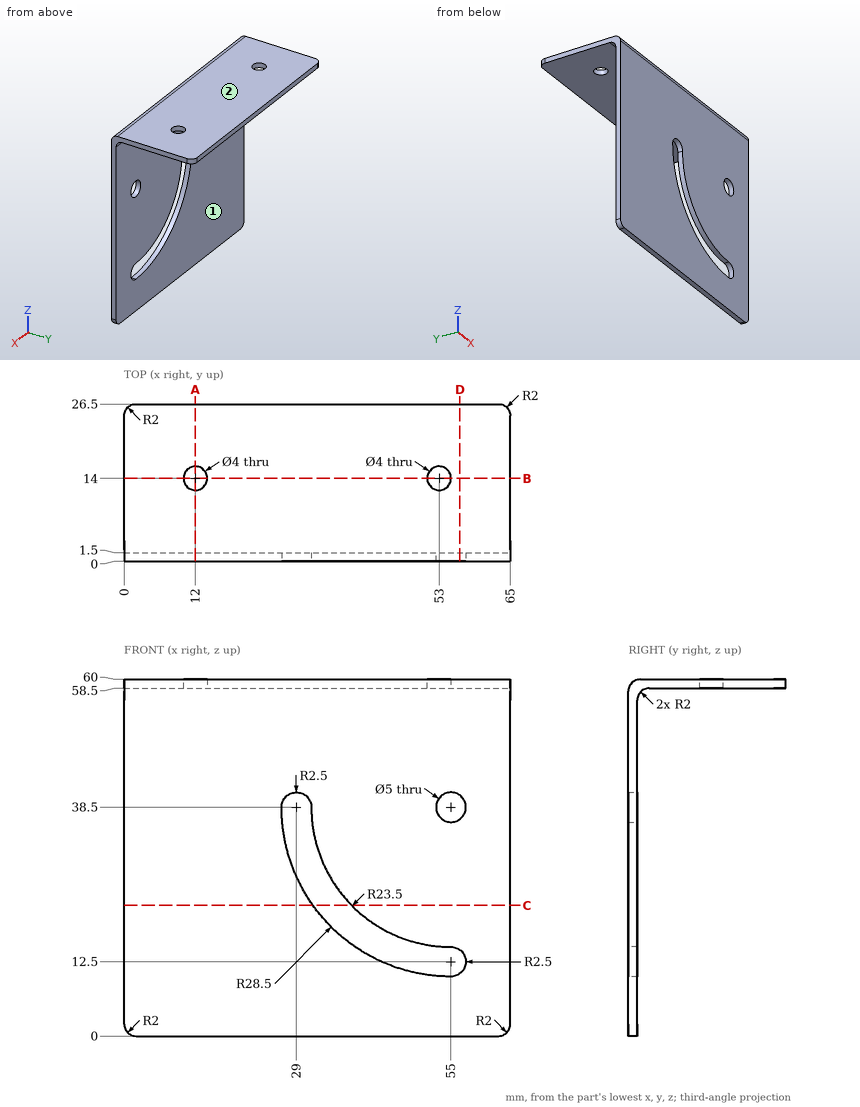
Verification items for this drawing (mm, ordinates from the low corner). A direction names the side the tool comes from. Coordinates: 2 decimals unless noted, no trailing zeros. Order: outer loops, then holes, each group sorted by start corner. A loop starts at its lowest first (then second) coordinate and runs counter-clockwise, first axis right, second up. Notation, with made-up numbers: (-23.5, 45.5) -> (26.5, 45.5) arc R15 cw to (26.5, 56.5) -> close; hole circle Ø3 at (47, -32). An arc over 180 degrees is marked (long way). Put each result on its own line as item: value. Start each with the question number.
1. Cross-section at B-B, the plane y = 14. Record the boundary of the cut face in (x, z).
2. Cross-section at C-C, the plane z = 22. Record the boundary of the cut face in (x, y), then the cut area to 3 significant figures.
3. Material ranges on L1, parallel to Z at x = 53, y = 10; L2, parallel to Y at x = 54, z = 7.5; L3, parallel to Z at x = 55, y = 0.9, recorded low to high. Write a range as [from, to].
4. Cross-section at D-D, the plane x = 56.5. Record the boundary of the cut face in (y, z).
5. Access from +Z, -Z, +X, -X, +Y, -Y to the whole of each face (thin tool, end or side, straight path). Record for the marked faces 1 and 2.
6. Go/stop test with flat-tipped pins: pin 1 Ø4 at (x, z) = (55, 38.5) entering from +Y; pin 2 Ø11.5 at (x, y) = (21, 11.5) entering from -Z. Record where each tip stops, or that it passes through.
7. Cross-section at A-A, the plane x = 12. Record the boundary of the cut face in (y, z).
Computed:
1. outline: (0, 58.5) -> (10, 58.5) -> (10, 60) -> (0, 60) -> close; (14, 58.5) -> (51, 58.5) -> (51, 60) -> (14, 60) -> close; (55, 58.5) -> (65, 58.5) -> (65, 60) -> (55, 60) -> close
2. outline: (0, 0) -> (31.76, 0) -> (31.76, 1.5) -> (0, 1.5) -> close; (38.27, 0) -> (65, 0) -> (65, 1.5) -> (38.27, 1.5) -> close
2. area: 87.7 mm2
3. L1: [58.5, 60]
3. L2: [0, 1.5]
3. L3: [0, 10], [15, 36], [41, 59.67]
4. outline: (0, 0) -> (1.5, 0) -> (1.5, 10.5) -> (0, 10.5) -> close; (0, 14.5) -> (1.5, 14.5) -> (1.5, 36.5) -> (0, 36.5) -> close; (0, 40.5) -> (1.5, 40.5) -> (1.5, 56.5) arc R2 cw to (3.5, 58.5) -> (26.5, 58.5) -> (26.5, 60) -> (2, 60) arc R2 ccw to (0, 58) -> close
5. face 1: -Z, +X, -X, +Y
5. face 2: +Z, +X, -X, +Y, -Y
6. pin 1: through
6. pin 2: z = 58.5
7. outline: (0, 0) -> (1.5, 0) -> (1.5, 56.5) arc R2 cw to (3.5, 58.5) -> (12, 58.5) -> (12, 60) -> (2, 60) arc R2 ccw to (0, 58) -> close; (16, 58.5) -> (26.5, 58.5) -> (26.5, 60) -> (16, 60) -> close
